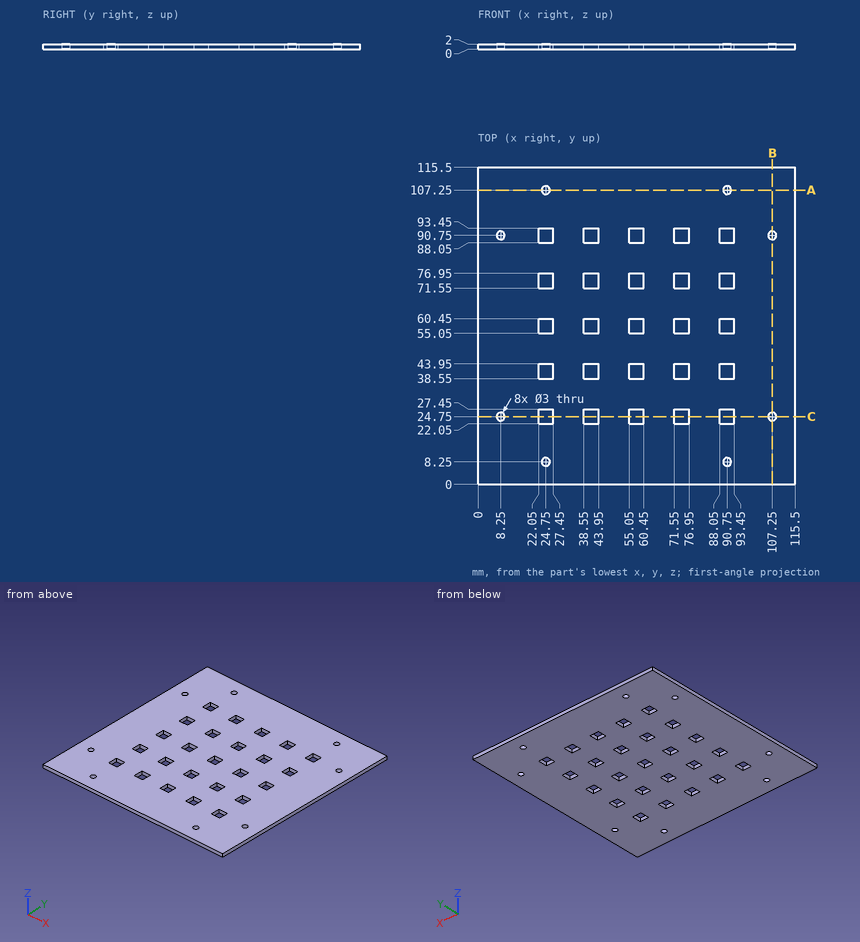
For this review, use the dimensioned drawing (mm, ordinates from the lowest corner) and the shaded views. Coordinates: 2 decimals unless noted, no trailing zeros. Order: outer loops, then holes, each group sorted by start corner. A loop starts at its lowest first (then second) coordinate and runs counter-clockwise, first axis right, second up. Notation, with made-up numbers: M 68.5,28 L 74.5,28 A23 ccw 74.5,58 Z; hole C 22,-9.5 d8. An arc over 180 degrees is marked long. Answer as a JSON object with one key per item and string values. Group by question number.
1) Add section C-C, the plane y = 24.75. Count the separate pieces of the cut face and the enclosed holes in it, then the cut area to 3 significant figures.
2) Wall thickness on L1, parallel to Y at x = 107.25, z = 0.7; L2, parallel to X at y = 58, z = 0.85: over which ranges is each line inside the solid? List them lowest first.
3) Add section A-A, the plane y = 107.25. Write out the cut boundary in (x, z), then the cut area to 3 significant figures.
Computed values:
{
 "1": {"separate pieces": "8", "enclosed holes": "0", "area": "165 mm^2"},
 "2": {"L1": "y = 0 to 23.25, 26.25 to 89.25, 92.25 to 115.5", "L2": "x = 0 to 22.05, 27.45 to 38.55, 43.95 to 55.05, 60.45 to 71.55, 76.95 to 88.05, 93.45 to 115.5"},
 "3": {"outline": "M 0,0 L 23.25,0 L 23.25,2 L 0,2 Z; M 26.25,0 L 89.25,0 L 89.25,2 L 26.25,2 Z; M 92.25,0 L 115.5,0 L 115.5,2 L 92.25,2 Z", "area": "219 mm^2"}
}
